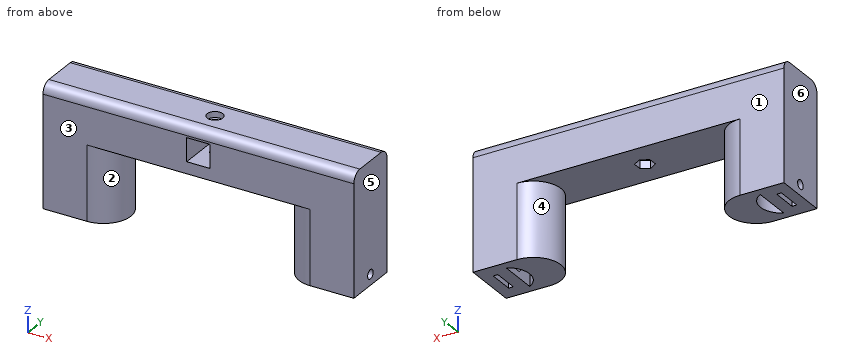
```python
from build123d import *

# Parameters (mm, degrees)
F0_W            = 12
F0_H            = 12
F1_DEPTH        = 28
F2_DEPTH        = 4
F3_W            = 2.4
F3_H            = 13
F4_DEPTH        = 13
F5_R            = 2.35
F6_DEPTH        = 14.5
F9_DEPTH        = 38
F11_D           = 4.8
F11_CBORE_D     = 8
F11_CBORE_DEPTH = 3
F12_DEPTH       = 4
F13_R           = 5


# Not quite as in the source:
# - a pattern or mirror of a feature is missing from the dataset's text; its kind, count and spacing are read off the source's solid


with BuildPart() as f1:
    # F0 (on Front) → F1 (new body)
    with BuildSketch(Plane.XZ):
        Polygon((0, 62), (0, 0), (14.5, 0), (14.5, 38), (144.5, 38), (144.5, 0), (159, 0), (159, 62), align=None)
        with Locations((79.5, 50)):
            Rectangle(F0_W, F0_H, mode=Mode.SUBTRACT)
    extrude(amount=F1_DEPTH)

    # F0 (on Front) → F2 (join)
    with BuildSketch(Plane.XZ):
        with Locations((79.5, 50)):
            Rectangle(F0_W, F0_H)
    extrude(amount=F2_DEPTH)

    # F3 (on face) → F4 (cut)
    with BuildSketch(Plane(origin=(0, 0, 0), x_dir=(1, 0, 0), z_dir=(0, 0, -1))):
        with Locations((7, 14)):
            Rectangle(F3_W, F3_H)
        with Locations((152, 14)):
            Rectangle(F3_W, F3_H)
    extrude(amount=-F4_DEPTH, mode=Mode.SUBTRACT)

    # F5 (on face) → F6 (cut)
    with BuildSketch(Plane(origin=(0, 0, 0), x_dir=(0, -1, 0), z_dir=(-1, 0, 0))):
        with Locations((14, 5.5)):
            Circle(F5_R)
    f6 = extrude(amount=-F6_DEPTH, mode=Mode.SUBTRACT)

    # F6_copies: F6 across plane
    add(f6.mirror(Plane(origin=(79.5, 0, 0), x_dir=(0, 0, 1), z_dir=(1, 0, 0))), mode=Mode.SUBTRACT)

    # F8 (on face) → F9 (join, through all)
    with BuildSketch(Plane(origin=(0, 0, 38), x_dir=(1, 0, 0), z_dir=(0, 0, -1))):
        with BuildLine():
            ThreePointArc((14.5, 24), (20.5, 14), (14.5, 4))
            Line((14.5, 4), (14.5, 0))
            Line((14.5, 0), (22.5, 0))
            ThreePointArc((22.5, 0), (36.5, 14), (22.5, 28))
            Line((22.5, 28), (14.5, 28))
            Line((14.5, 28), (14.5, 24))
        make_face()
    f9 = extrude(amount=F9_DEPTH)

    # F9_copies: F9 across plane
    add(f9.mirror(Plane(origin=(79.5, 0, 0), x_dir=(0, 0, 1), z_dir=(1, 0, 0))))

    # F11 (through all)
    with Locations(Plane.XY.offset(62)):
        with Locations((79.5, -14)):
            CounterBoreHole(F11_D / 2, F11_CBORE_D / 2, F11_CBORE_DEPTH)

    # F8 (on face) → F12 (cut)
    with BuildSketch(Plane(origin=(0, 0, 38), x_dir=(1, 0, 0), z_dir=(0, 0, -1))):
        Polygon((79.5955098336, 9.4009916426), (83.5306129865, 11.7832097635), (83.4351031529, 16.3822181209), (79.4044901664, 18.5990083574), (75.4693870135, 16.2167902365), (75.5648968471, 11.6177818791), align=None)
    extrude(amount=-F12_DEPTH, mode=Mode.SUBTRACT)

    # F13
    f13_edges = [f1.edges().sort_by_distance(p)[0] for p in [
        (79.5, -28, 62),
        (79.5, 0, 62),
    ]]
    fillet(f13_edges, radius=F13_R)


solid = f1.part
```
Check sheet for the modelled part. Datum: model origin and axes. Units: mm. Face numbers are marked on the shaded views. A direction names the side the tool comes from. Coordinates: 2 decimals unless noted, no trailing zeros. Loops run counter-clockwise (first coordinate to the right, second up) from the corner with the lowest first, then second, coordinate; pieces in that order, holes last.
1) Sectioned sample at C-C (x = 141). Record the boundary of the cut face in (y, z), and give its area (3 significant figures).
2) Sectioned sample at D-D (y = -14). Count the separate pieces of the cut face and the enclosed holes in it, and give its area (3 significant figures).
3) Access from +Z, -Z, +X, -X, +Y, -Y to the whole of each face (thin tool, end or side, straight path). Record for the marked faces 1 and 2.
4) Material ranges on probe 1 along X at (y, z) = (-14, 26.5); probe 2 along Y at (x, z) = (79.5, 57.4); probe 3 along Z at (x, y) = (11.25, -14), recorded low to high.
5) Release check for a two-part mould opening along X. For the marked faces 3, 4, 5 and 6 record: released by +X, released by -X, zero draft, split by the parting line, or undercut.
6) Gauge pin test, flat ends, axial feed: pin 1 (1.8 mm diameter, centred on x = 19, y = -13, fed in from -Z); pin 2 (4 mm diameter, centred on x = 80.5, y = -12.5, fed in from -Z); pin 3 (6.5 mm diameter, centred on x = 79.5, y = -14, fed in from +Z). Record the tip position at first contact, or that the pin passes through.
7) Sectioned sample at A-A (z = 33). Record the boundary of the cut face in (x, y).
8) Sectioned sample at B-B (z = 49.5). Record the boundary of the cut face in (x, y), and give its area (3 significant figures).
Check sheet entries:
1. outline: (-28, 0) - (-21.1, 0) - (-21.1, 38) - (-6.9, 38) - (-6.9, 0) - (0, 0) - (0, 57) arc R5 ccw to (-5, 62) - (-23, 62) arc R5 ccw to (-28, 57) - close
1. area: 1,190 mm2
2. separate pieces: 6
2. enclosed holes: 0
2. area: 5,730 mm2
3. face 1: +Z, -Z, +X, -X, +Y
3. face 2: -Z
4. probe 1: x = 0 to 14.5, 20.5 to 36.5, 122.5 to 138.5, 144.5 to 159
4. probe 2: y = -27.98 to -16.4, -11.6 to -0.02
4. probe 3: z = 0 to 3.15, 7.85 to 62
5. face 3: zero draft
5. face 4: undercut
5. face 5: released by +X
5. face 6: released by -X
6. pin 1: stops at z = 38
6. pin 2: stops at z = 42
6. pin 3: stops at z = 59
7. outline: (0, -28) - (22.5, -28) arc R14 ccw to (22.5, 0) - (0, 0) - close; (136.5, -28) - (159, -28) - (159, 0) - (136.5, 0) arc R14 ccw to start; hole (14.5, -24) arc R11.33 ccw to (14.5, -4) - close; hole (144.5, -24) - (144.5, -4) arc R11.33 ccw to start
8. outline: (0, -28) - (73.5, -28) - (73.5, -4) - (85.5, -4) - (85.5, -28) - (159, -28) - (159, 0) - (0, 0) - close
8. area: 4,160 mm2
